Could you check a few things on this drawing? It's one solid part, dimensions in mm from its lowest x, y, z. A direction names the side the tool comes from. Give positions to 0.01 mm unless a question says otherwise; leave off trailing zeros. Order: outer loops, then holes, each group sorted by start corner. A loop starts at its lowest first (then second) coordinate and runs counter-clockwise, first axis right, second up.
Item 1: I'm going to push flat-ended pins straight in: pin 1 Ø8 at (y, z) = (10, 40) entering from -X; pin 2 Ø7 at (x, y) = (40, 10) entering from +Z; pin 3 Ø8 at (y, z) = (8, 12.5) entering from -X; pin 4 Ø5 at (y, z) = (10, 40) entering from +X. Where does each tip first touch, or does it pass through?
Item 2: I want a section at B-B, the plane z = 12. Write out the boundary of the cut face in (x, y).
Item 3: I want a section at C-C, the plane x = 4.5. Write out the boundary of the cut face in (y, z), then the cut area to 3 significant figures.
Item 4: If I drill on line 1 along Y through (x, z) = (40, 47); line 2 along Y through (x, z) = (40, 4.1); line 3 along Z through (x, y) = (8.5, 18.75), over which ranges is the centre line in solid material (lowest first)?
Item 5: I want a section at A-A, the plane y = 10. Count the separate pieces of the cut face and the enclosed holes in it, then the cut area to 3 significant figures.
Item 6: If we mould it in two halves opening along X, with no side actions, what happens to the marked faces 1, 2 and 3? For each: +X half, -X half, draft (parallel to the pull), parting line (faces both ways), or undercut.
Item 7: I want a section at D-D, the plane y = 18.75. Write out the boundary of the cut face in (x, z).
Item 8: Which directions (+Z, -Z, +X, -X, +Y, -Y) give clear straight access to the entire face, cutting with the end or side of a thin tool? Please do the marked faces 4, 5 and 6.
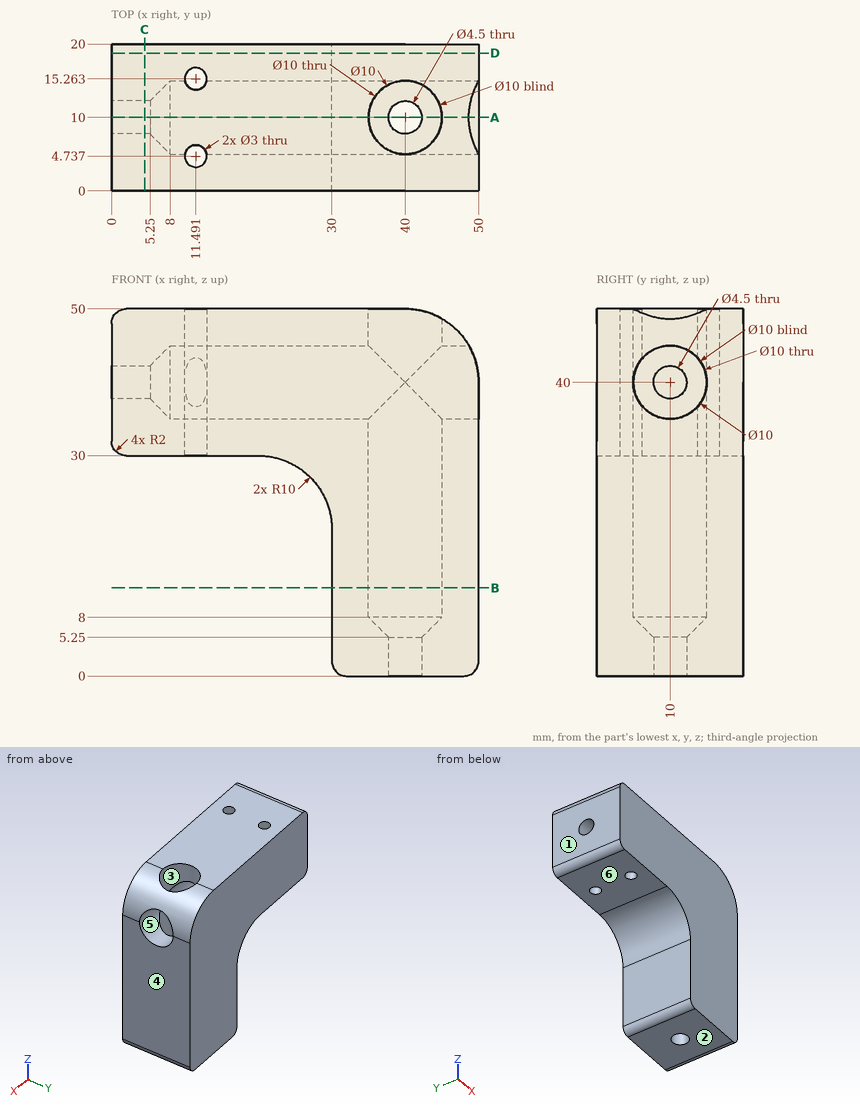
Results list:
1. pin 1: stops at x = 0
1. pin 2: stops at z = 6.5
1. pin 3: stops at x = 30
1. pin 4: stops at x = 5.5
2. outline: (30, 0) - (50, 0) - (50, 20) - (30, 20) - close; hole circle Ø10 at (40, 10)
3. outline: (0, 30) - (20, 30) - (20, 50) - (0, 50) - close; hole circle Ø4.5 at (10, 40)
3. area: 384 mm2
4. line 1: y = 0 to 5, 15 to 20
4. line 2: y = 0 to 7.75, 12.25 to 20
4. line 3: z = 30 to 50
5. separate pieces: 4
5. enclosed holes: 0
5. area: 774 mm2
6. face 1: -X half
6. face 2: draft
6. face 3: undercut
7. outline: (0, 32) arc R2 ccw to (2, 30) - (20, 30) arc R10 cw to (30, 20) - (30, 2) arc R2 ccw to (32, 0) - (48, 0) arc R2 ccw to (50, 2) - (50, 40) arc R10 ccw to (40, 50) - (2, 50) arc R2 ccw to (0, 48) - close
8. face 4: +Z, -Z, +X, +Y, -Y
8. face 5: +X
8. face 6: -Z, -X, +Y, -Y
